Check sheet for the modelled part. Datum: model origin and axes. Units: mm. Give positions to 0.01 mm unless a question says otherwise; leave off trailing zeros. Loops run counter-clockwise (first coordinate to the right, second up) from the corner with the lowest first, then second, coordinate; pieces in that order, holes last. Notation, with made-up numbers: (88.5, 24.25) -> (119.5, 24.25) arc R37 cw to (119.5, 60.25) -> close; hole circle Ø8 at (24.5, 52.25). An arc over 180 degrees is marked (long way). Write each question's results on one line, items separated by ' | '. Start each with the question number.
1. Cross-section at B-B on y = 0.55. Count the separate pieces of the cut face and the enclosed holes in it, and give its area (3 significant figures).
2. Material ranges on L1, parallel to X at y = 0.4, z = -60 (3 decimals); L2, parallel to Z at x = 3.5, y = 0.9 (3 decimals); L3, parallel to X at y = 0.65, z = -73.5, recorded low to high. Write a range as from..to.
3. Cross-section at A-A on x = 106.5. Record the boundary of the cut face in (y, z) (3 decimals).
4. Mould release check, pull along X, two halves, no side actions. Record for faces 1 (the face through (54, 0, -46)), 2 (the face through (3.09, 0.89, -43.14)): +X half, -X half, draft (parallel to the pull), parting line (faces both ways), or undercut.
5. Gauge pin test, flat ends, axial feed: pin 1 Ø3 at (x, z) = (106.5, -75) entering from -Y; pin 2 Ø0.5 at (x, y) = (56.5, 1.5) entering from -Z. Record the tip position at first contact, or that the pin passes through.
6. Cross-section at C-C on z = -75. Record the boundary of the cut face in (x, y) (3 decimals).
from build123d import *

# Parameters (mm, degrees)
FR4_DEPTH          = 1.7526
SKETCH7_R          = 1.905
CUT_EXTRUDE1_DEPTH = 2.7526


with BuildPart() as part:
    # Sketch1 → FR4 (new body)
    with BuildSketch(Plane(origin=(0, 0, 0), x_dir=(1, 0, 0), z_dir=(0, 1, 0))):
        with BuildLine():
            Line((0, 0), (110, 0))
            Line((110, 0), (110, 87))
            Line((110, 87), (104, 87))
            ThreePointArc((104, 87), (102.585786438, 87.585786438), (102, 89))
            Line((102, 89), (102, 90))
            Line((102, 90), (64, 90))
            Line((64, 90), (64, 89))
            ThreePointArc((64, 89), (63.414213562, 87.585786438), (62, 87))
            Line((62, 87), (48, 87))
            ThreePointArc((48, 87), (46.585786438, 87.585786438), (46, 89))
            Line((46, 89), (46, 90))
            Line((46, 90), (8, 90))
            Line((8, 90), (8, 89))
            ThreePointArc((8, 89), (7.414213562, 87.585786438), (6, 87))
            Line((6, 87), (0, 87))
            Line((0, 87), (0, 0))
        make_face()
    extrude(amount=FR4_DEPTH)

    # Sketch7 → Cut-Extrude1 (cut, through all)
    with BuildSketch(Plane(origin=(0, 1.7526, 0), x_dir=(1, 0, 0), z_dir=(0, 1, 0))):
        with Locations((3.5, 15)):
            Circle(SKETCH7_R)
        with Locations((106.5, 15)):
            Circle(SKETCH7_R)
        with Locations((106.5, 30)):
            Circle(SKETCH7_R)
        with Locations((106.5, 45)):
            Circle(SKETCH7_R)
        with Locations((106.5, 60)):
            Circle(SKETCH7_R)
        with Locations((106.5, 75)):
            Circle(SKETCH7_R)
        with Locations((3.5, 30)):
            Circle(SKETCH7_R)
        with Locations((3.5, 45)):
            Circle(SKETCH7_R)
        with Locations((3.5, 60)):
            Circle(SKETCH7_R)
        with Locations((3.5, 75)):
            Circle(SKETCH7_R)
    extrude(amount=-CUT_EXTRUDE1_DEPTH, mode=Mode.SUBTRACT)


solid = part.part
Geometry says:
1) separate pieces: 1 | enclosed holes: 10 | area: 9,690 mm^2
2) L1: 0..1.595, 5.405..104.595, 108.405..110 | L2: -87..-76.905, -73.095..-61.905, -58.095..-46.905, -43.095..-31.905, -28.095..-16.905, -13.095..0 | L3: 0..2.33, 4.67..105.33, 107.67..110
3) outline: (0, -87) -> (1.753, -87) -> (1.753, -76.905) -> (0, -76.905) -> close; (0, -73.095) -> (1.753, -73.095) -> (1.753, -61.905) -> (0, -61.905) -> close; (0, -58.095) -> (1.753, -58.095) -> (1.753, -46.905) -> (0, -46.905) -> close; (0, -43.095) -> (1.753, -43.095) -> (1.753, -31.905) -> (0, -31.905) -> close; (0, -28.095) -> (1.753, -28.095) -> (1.753, -16.905) -> (0, -16.905) -> close; (0, -13.095) -> (1.753, -13.095) -> (1.753, 0) -> (0, 0) -> close
4) face 1: draft | face 2: undercut
5) pin 1: through | pin 2: z = -87
6) outline: (0, 0) -> (1.595, 0) -> (1.595, 1.753) -> (0, 1.753) -> close; (5.405, 0) -> (104.595, 0) -> (104.595, 1.753) -> (5.405, 1.753) -> close; (108.405, 0) -> (110, 0) -> (110, 1.753) -> (108.405, 1.753) -> close
